Source: three-view drawing plus pictorial views. Frame: mm from the lowest corner of the part. A direction names the side the tool comes from. Give positions to 0.01 mm unless a question says otherwise; leave off trailing zeros. Loops run counter-clockwise (first coordinate to the right, second up) from the corner with the lowest first, then second, coordinate; pieces in that order, holes last. Notation, with made-up numbers: (89, 71) -> (97, 71) arc R25 cw to (97, 85) -> close; hole circle Ø10 at (5, -28). An arc over 180 degrees is marked (long way). One line per item, written item: value. Start each with the question number.
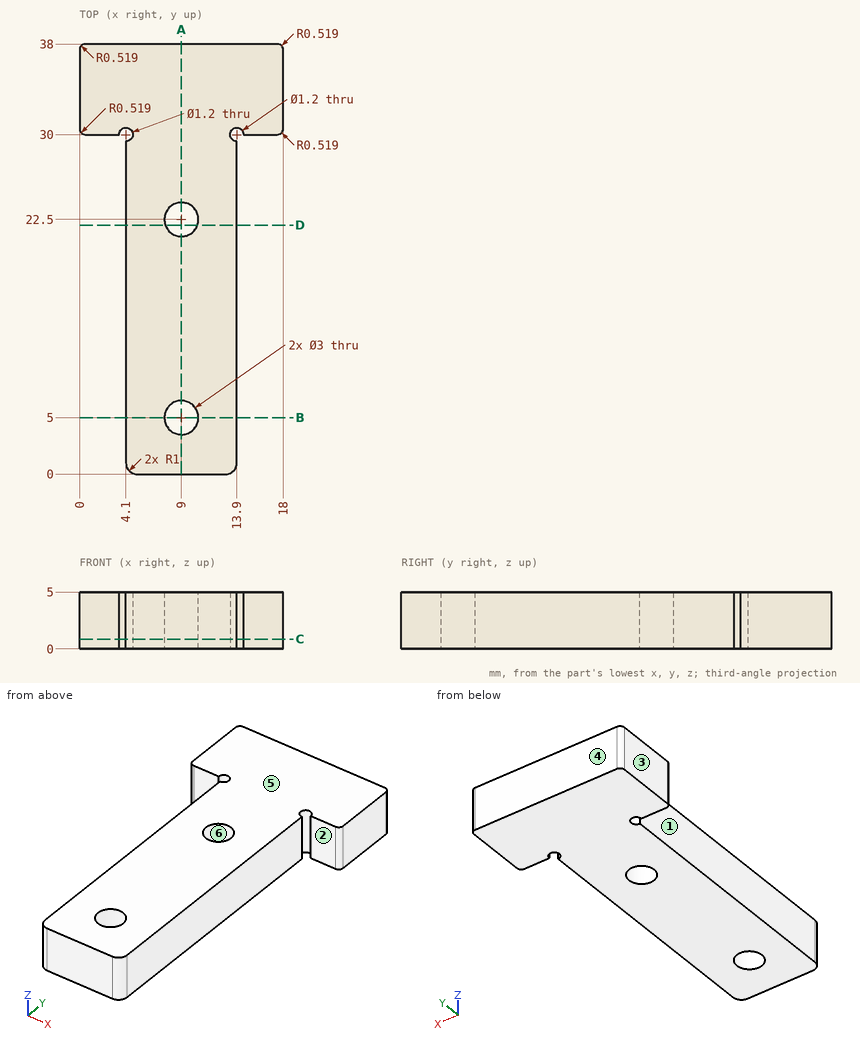
Item 1: Section C-C, the plane z = 0.85. Output: boundary loops of the cut face in (x, y).
Item 2: Section A-A, the plane x = 9. Output: boundary loops of the cut face in (y, z).
Item 3: Pin query (flat end, axial travel): pin 1 (1.5 mm diameter, centred on y = 17, z = 1.5, fed in from +X); pin 2 (2.5 mm diameter, centred on x = 2, z = 1.5, fed in from -Y); pin 3 (2.5 mm diameter, centred on y = 18, z = 1.5, fed in from -X). Return the tip coordinate at first contact, or that it passes through.
Item 4: Access query for the marked faces 1, 2 and 3. Directions: +Z, -Z, +X, -X, +Y, -Y. A direction counts if a zero-diameter tool reaches every point of the face in a straight line with its end or side. Return the directions, or none.
Item 5: Ray query, line 1 along Y through (x, z) = (9, 2.35); line 2 along Y through (x, z) = (8.5, 0.95) (1 decimal); line 3 along X through (y, z) = (10.5, 3.65). Return the intervals inside material, ascending. Write a range as [from, to].
Item 6: Mould query, pull axis Y, two halves, no side actions, for the marked faces 4, 5 and 6. Classes: pulls with the +Y half, pulls with the -Y half, needs draft (parallel to the pull), parting line crosses it, or undercut.
Item 7: Section D-D, the plane y = 22. Output: boundary loops of the cut face in (x, z) (1 decimal).
Item 8: Section B-B, the plane y = 5. Output: boundary loops of the cut face in (x, z).
Geometry check:
1. outline: (0, 30.52) arc R0.52 ccw to (0.52, 30) -> (3.5, 30) arc R0.6 cw (long way) to (4.1, 29.4) -> (4.1, 1) arc R1 ccw to (5.1, 0) -> (12.9, 0) arc R1 ccw to (13.9, 1) -> (13.9, 29.4) arc R0.6 cw (long way) to (14.5, 30) -> (17.48, 30) arc R0.52 ccw to (18, 30.52) -> (18, 37.48) arc R0.52 ccw to (17.48, 38) -> (0.52, 38) arc R0.52 ccw to (0, 37.48) -> close; hole circle Ø3 at (9, 5); hole circle Ø3 at (9, 22.5)
2. outline: (0, 0) -> (3.5, 0) -> (3.5, 5) -> (0, 5) -> close; (6.5, 0) -> (21, 0) -> (21, 5) -> (6.5, 5) -> close; (24, 0) -> (38, 0) -> (38, 5) -> (24, 5) -> close
3. pin 1: stops at x = 13.9
3. pin 2: stops at y = 30
3. pin 3: stops at x = 4.1
4. face 1: +Z, -Z, -X, -Y
4. face 2: +Z, -Z, +X, -Y
4. face 3: +Z, -Z, -X, +Y, -Y
5. line 1: y = [0, 3.5], [6.5, 21], [24, 38]
5. line 2: y = [0, 3.6], [6.4, 21.1], [23.9, 38]
5. line 3: x = [4.1, 13.9]
6. face 4: pulls with the +Y half
6. face 5: needs draft
6. face 6: undercut
7. outline: (4.1, 0) -> (7.6, 0) -> (7.6, 5) -> (4.1, 5) -> close; (10.4, 0) -> (13.9, 0) -> (13.9, 5) -> (10.4, 5) -> close
8. outline: (4.1, 0) -> (7.5, 0) -> (7.5, 5) -> (4.1, 5) -> close; (10.5, 0) -> (13.9, 0) -> (13.9, 5) -> (10.5, 5) -> close
